from build123d import *

# Parameters (mm, degrees)
SKETCH1_W           = 20
SKETCH1_H           = 40
BOSS_EXTRUDE1_DEPTH = 0.78
SKETCH4_W           = 6
SKETCH4_H           = 7.65
BOSS_EXTRUDE2_DEPTH = 6
SKETCH4_3_R         = 3
BOSS_EXTRUDE3_DEPTH = 7.6
SKETCH5_W           = 7.8
SKETCH5_H           = 5.4
BOSS_EXTRUDE4_DEPTH = 3
SKETCH6_W           = 16
SKETCH6_H           = 12.2
BOSS_EXTRUDE5_DEPTH = 2.4


with BuildPart() as part:
    # Sketch1 → Boss-Extrude1 (new body)
    with BuildSketch(Plane(origin=(0, 0, 0), x_dir=(1, 0, 0), z_dir=(0, 1, 0))):
        with Locations((0, -20)):
            Rectangle(SKETCH1_W, SKETCH1_H)
    extrude(amount=BOSS_EXTRUDE1_DEPTH)

    # Sketch4 → Boss-Extrude2 (add)
    with BuildSketch(Plane.XY):
        with Locations((6.25, 4.605)):
            Rectangle(SKETCH4_W, SKETCH4_H)
    extrude(amount=BOSS_EXTRUDE2_DEPTH)

    # Sketch4<3> → Boss-Extrude3 (add)
    with BuildSketch(Plane.XY):
        with Locations((6.25, 5.43)):
            Circle(SKETCH4_3_R)
    extrude(amount=-BOSS_EXTRUDE3_DEPTH)

    # Sketch5 → Boss-Extrude4 (add)
    with BuildSketch(Plane(origin=(0, 0.78, 0), x_dir=(1, 0, 0), z_dir=(0, 1, 0))):
        with Locations((5.35, -37.3)):
            Rectangle(SKETCH5_W, SKETCH5_H)
    extrude(amount=BOSS_EXTRUDE4_DEPTH)

    # Sketch6 → Boss-Extrude5 (add)
    with BuildSketch(Plane(origin=(0, 0.78, 0), x_dir=(1, 0, 0), z_dir=(0, 1, 0))):
        with Locations((0, -14.432954473)):
            Rectangle(SKETCH6_W, SKETCH6_H)
    extrude(amount=BOSS_EXTRUDE5_DEPTH)


solid = part.part
Geometry: final body of the model. Coordinates: model frame, mm. A direction names the side the tool comes from. Coordinates: 2 decimals unless noted, no trailing zeros. Order: outer loops, then holes, each group sorted by start corner. A loop starts at its lowest first (then second) coordinate and runs counter-clockwise, first axis right, second up. Notation, with made-up numbers: M 77.5,-31 L 132.5,-31 A14 ccw 132.5,-13 Z; hole C 52,-8 d5. An arc over 180 degrees is marked long. One line per question, with ' | ' between items. Start each with the question number.
Item 1: Ray query, probe 1 along Z at (x, y) = (3.5, 1); probe 2 along Y at (x, z) = (-0.75, 16); probe 3 along X at (y, z) = (7.5, 5.5). Return the intervals inside material, ascending. Write a range as [from, to].
Item 2: Set-up query: faces 1 (the flat face through (0, 2, 20.533)), 2 (the flat face through (9.25, 2, 37)), 3 (the flat face through (9, 8, 0)), 4 (the flat face through (-8, 2, 15)). Return all of +Z, -Z, +X, -X, +Y, -Y with unobstructed straight access to the full face (end or side cutting, diameter ignored); none if empty.
Item 3: Draft query along Z for faces 5 (the flat face through (4, 1, 40)), 6 (the flat face through (6, 5, 6)), 7 (the flat face through (8, 2, 15)), 8 (the flat face through (5, 3.78, 37)). Return one class per face: released by +Z, released by -Z, zero draft, split by the parting line, or undercut.
Item 4: Cut plane A-A, the plane y = 2. Return the cut outline in (x, z).
Item 5: Cut plane B-B, the plane z = 4. Return the cut outline in (x, y).
Item 6: Pin query (flat end, axial travel): pin 1 Ø5 at (y, z) = (5.5, 3) entering from -X; pin 2 Ø10 at (x, z) = (1, 15) entering from +Y; pin 3 Ø0.9 at (y, z) = (2.5, 36) entering from -X; pin 4 Ø4 at (x, y) = (0, 7.5) entering from +Z. Return the tip coordinate at first contact, or that it passes through.
Item 7: Cut plane C-C, the plane x = -7. Return the cut outline in (y, z), then the cut area to 3 significant figures.
Item 8: Cut plane D-D, the plane x = 4.75. Return the cut outline in (y, z), then the cut area to 3 significant figures.
A:
1) probe 1: z = [0, 6], [8.33, 20.53], [34.6, 40] | probe 2: y = [0, 3.18] | probe 3: x = [3.25, 9.25]
2) face 1: +X, -X, +Y | face 2: +Z, -Z, +X, +Y | face 3: -Z, +X, +Y | face 4: +Z, -Z, -X, +Y
3) face 5: released by +Z | face 6: undercut | face 7: undercut | face 8: zero draft
4) outline: M -8,8.33 L 8,8.33 L 8,20.53 L -8,20.53 Z; M 1.45,34.6 L 9.25,34.6 L 9.25,40 L 1.45,40 Z; M 3.25,0 L 9.25,0 L 9.25,6 L 3.25,6 Z
5) outline: M -10,0 L 10,0 L 10,0.78 L 9.25,0.78 L 9.25,8.43 L 3.25,8.43 L 3.25,0.78 L -10,0.78 Z
6) pin 1: stops at x = 3.25 | pin 2: stops at y = 3.18 | pin 3: stops at x = 1.45 | pin 4: passes through
7) outline: M 0,0 L 0.78,0 L 0.78,8.33 L 3.18,8.33 L 3.18,20.53 L 0.78,20.53 L 0.78,40 L 0,40 Z | area: 60.5 mm2
8) outline: M 0,0 L 2.83,0 L 2.83,-7.6 L 8.03,-7.6 L 8.03,0 L 8.43,0 L 8.43,6 L 0.78,6 L 0.78,8.33 L 3.18,8.33 L 3.18,20.53 L 0.78,20.53 L 0.78,34.6 L 3.78,34.6 L 3.78,40 L 0,40 Z | area: 162 mm2
